Work out the finished part from the listing and answer in its coordinate system (mm). A direction names the side the tool comes from. Round coordinates to 2 decimals unless told otherwise and drop trailing zeros. Write each loop counter-clockwise with the first axis right and the second up, starting at its lowest first coordinate (ties: lowest second). Pieces come first, ordered by that corner, then holes. Notation, with made-up numbers: M 75.25,11.25 L 130.25,11.25 A19 ccw 130.25,22.25 Z; hole C 51.5,-27.5 d4. An arc over 180 degrees is marked long. One line per item, written item: value. Start each with the question number.
Q1. Find section D-D (x = 41). Write down the section's boundary in (y, z), and give its area (3 significant figures).
Q2. Find section B-B (y = 0.9). Write down the section's boundary in (x, z), and give its area (3 significant figures).
Q3. Find section A-A (x = 2.35). Write down the section's boundary in (y, z), and give its area (3 significant figures).
Q4. Consider probe 1 along X at (y, z) = (0.45, -53.65); probe 2 along Z at (x, y) = (2.35, 0.45); probe 3 along X at (y, z) = (0.8, -4.5). Determine where each line is inside the solid, lowest interval first.
Q5. A tool of negligible diameter and unlimited length cuts with its end or side. For faces 1 (the flat face through (35, 1, -6)), 2 (the flat face through (35, 1, -56)), from which of +Z, -Z, +X, -X, +Y, -Y can it reach the whole face along a straight path? Write none if from no direction.
Q6. Given pin 1 Ø6 at (x, z) = (12, -26) entering from -Y; pin 2 Ø1.8 at (x, z) = (68.65, -53.65) entering from -Y, each flat-ended and moving along its own axis, determine where each tip first touches the part or whether it passes through.
Q7. The mould has two halves that part along X. Classify faces 3 (the flat face through (35, 1.5, -28)), 4 (the flat face through (71, 1, -28)), 5 (the cylindrical face through (2.112, 0.76, -52.576)), 6 (the flat face through (0, 1, -28)): released by +X, released by -X, zero draft, split by the parting line, or undercut.
Q8. Find section C-C (z = -2.35). Write down the section's boundary in (x, y), and give its area (3 significant figures).
from build123d import *

# Parameters (mm, degrees)
SKETCH1_W           = 71
SKETCH1_H           = 56
BOSS_EXTRUDE1_DEPTH = 1.5
SKETCH2_W           = 20
SKETCH2_H           = 6
CUT_EXTRUDE1_DEPTH  = 1.5
SKETCH5_R           = 1.1
CUT_EXTRUDE2_DEPTH  = 1.5


with BuildPart() as part:
    # Sketch1 → Boss-Extrude1 (new body)
    with BuildSketch(Plane(origin=(0, 0, 0), x_dir=(1, 0, 0), z_dir=(0, 1, 0))):
        with Locations((35.5, 28)):
            Rectangle(SKETCH1_W, SKETCH1_H)
    extrude(amount=BOSS_EXTRUDE1_DEPTH)

    # Sketch2 → Cut-Extrude1 (cut)
    with BuildSketch(Plane(origin=(0, 1.5, 0), x_dir=(1, 0, 0), z_dir=(0, 1, 0))):
        with Locations((35.5, 3)):
            Rectangle(SKETCH2_W, SKETCH2_H)
    extrude(amount=-CUT_EXTRUDE1_DEPTH, mode=Mode.SUBTRACT)

    # Sketch5 → Cut-Extrude2 (cut)
    with BuildSketch(Plane(origin=(0, 1.5, 0), x_dir=(1, 0, 0), z_dir=(0, 1, 0))):
        with Locations((2.35, 53.65)):
            Circle(SKETCH5_R)
        with Locations((68.65, 53.65)):
            Circle(SKETCH5_R)
    cut_extrude2 = extrude(amount=-CUT_EXTRUDE2_DEPTH, mode=Mode.SUBTRACT)

    # Mirror1: Cut-Extrude2 across plane
    add(cut_extrude2.mirror(Plane.XY.offset(-28)), mode=Mode.SUBTRACT)


solid = part.part
The answers:
1. outline: M 0,-56 L 1.5,-56 L 1.5,-6 L 0,-6 Z
1. area: 75.0 mm2
2. outline: M 0,-56 L 71,-56 L 71,0 L 45.5,0 L 45.5,-6 L 25.5,-6 L 25.5,0 L 0,0 Z; hole C 2.35,-53.65 d2.2; hole C 2.35,-2.35 d2.2; hole C 68.65,-53.65 d2.2; hole C 68.65,-2.35 d2.2
2. area: 3,840 mm2
3. outline: M 0,-56 L 1.5,-56 L 1.5,-54.75 L 0,-54.75 Z; M 0,-52.55 L 1.5,-52.55 L 1.5,-3.45 L 0,-3.45 Z; M 0,-1.25 L 1.5,-1.25 L 1.5,0 L 0,0 Z
3. area: 77.4 mm2
4. probe 1: 0 to 1.25, 3.45 to 67.55, 69.75 to 71
4. probe 2: -56 to -54.75, -52.55 to -3.45, -1.25 to 0
4. probe 3: 0 to 25.5, 45.5 to 71
5. face 1: +Z, +Y, -Y
5. face 2: -Z, +X, -X, +Y, -Y
6. pin 1: y = 0
6. pin 2: through
7. face 3: zero draft
7. face 4: released by +X
7. face 5: undercut
7. face 6: released by -X
8. outline: M 0,0 L 1.25,0 L 1.25,1.5 L 0,1.5 Z; M 3.45,0 L 25.5,0 L 25.5,1.5 L 3.45,1.5 Z; M 45.5,0 L 67.55,0 L 67.55,1.5 L 45.5,1.5 Z; M 69.75,0 L 71,0 L 71,1.5 L 69.75,1.5 Z
8. area: 69.9 mm2
